Verification items for the finished model (mm, model axes). A direction names the side the tool comes from. Coordinates: 2 decimals unless noted, no trailing zeros. Order: outer loops, then holes, each group sorted by start corner. A loop starts at its lowest first (then second) coordinate and runs counter-clockwise, first axis right, second up. Notation, with made-up numbers: M -13.75,40 L 36.25,40 A14 cw 36.25,55 Z; hole C 53,75 d9. An arc over 180 degrees is marked long. Answer as a JSON object with one key per item and string values. Group by question number.
(1) Access from +Z, -Z, +X, -X, +Y, -Y to the whole of each face (thin tool, end or side, straight path). Record for faces 4 (the face through (38.1, -11, 37)), 5 (the face through (19, -14, 63.5)), 6 (the face through (39.39, -19.54, 53.44)).
(2) Mould release check, pull along Y, two halves, no side actions. Record for faces 1 (the face through (39.39, -6.84, 53.44)), 2 (the face through (-1.776, -0.724, 30.053)), 3 (the face through (-2.54, -14, 30)): released by +Y, released by -Y, zero draft, split by the parting line, or undercut.
(3) Material ranges on line 1 (X direction, y = -15.5, z = 17.5); line 2 (Y direction, x = 38.7, z = 54.61); line 3 (Y direction, x = 39, z = 54), recorded low to high.
(4) Cross-section at D-D (y = -6.35). Enter the section's corners in (x, z).
(5) Cross-section at A-A (z = 54.61). Count the separate pieces of the cut face and the enclosed holes in it, plus the area to 3 significant figures.
(6) Gauge pin test, flat ends, axial feed: pin 1 Ø1 at (x, z) = (23.5, 36) entering from +Y; pin 2 Ø7 at (x, y) = (14.5, -13.5) entering from -Z; pin 3 Ø4 at (x, y) = (19, -22.5) entering from -Z. Record the tip position at first contact, or that the pin passes through.
from build123d import *

# Parameters (mm, degrees)
BOSS_EXTRUDE2_DEPTH = 38.1
BOSS_EXTRUDE3_DEPTH = 2.54
BOSS_EXTRUDE5_START = 2.54
BOSS_EXTRUDE5_DEPTH = 2.54
FILLET1_R           = 2.54
FILLET3_R           = 2.54
FILLET5_R           = 2.54
SKETCH5_R           = 1.27
CUT_EXTRUDE1_DEPTH  = 2.54


with BuildPart() as part:
    # Sketch1 → Boss-Extrude2 (new body)
    with BuildSketch(Plane(origin=(0, 0, 0), x_dir=(0, 0, -1), z_dir=(1, 0, 0))):
        with BuildLine():
            Line((-60.96, 0), (-63.5, 0))
            Line((-63.5, 0), (-63.5, -25.4))
            Line((-63.5, -25.4), (-25.4, -25.4))
            ThreePointArc((-25.4, -25.4), (-7.439487758, -17.960512242), (0, 0))
            Line((0, 0), (-2.681549349, -2.54))
            ThreePointArc((-2.681549349, -2.54), (-10.16, -17.038837989), (-25.4, -22.86))
            Line((-25.4, -22.86), (-60.96, -22.86))
            Line((-60.96, -22.86), (-60.96, 0))
        make_face()
    extrude(amount=BOSS_EXTRUDE2_DEPTH)

    # Sketch2 → Boss-Extrude3 (add)
    with BuildSketch(Plane(origin=(38.1, 0, 0), x_dir=(0, 0, -1), z_dir=(1, 0, 0))):
        with BuildLine():
            Line((-63.5, 0), (0, 0))
            ThreePointArc((0, 0), (-7.439487758, -17.960512242), (-25.4, -25.4))
            Line((-25.4, -25.4), (-63.5, -25.4))
            Line((-63.5, -25.4), (-63.5, 0))
        make_face()
    extrude(amount=BOSS_EXTRUDE3_DEPTH)

    # Sketch3 → Boss-Extrude5 (add)
    with BuildSketch(Plane.ZY.offset(BOSS_EXTRUDE5_START)):
        with BuildLine():
            Line((2.681549349, -2.54), (0, 0))
            ThreePointArc((0, 0), (7.439487758, -17.960512242), (25.4, -25.4))
            Line((25.4, -25.4), (63.5, -25.4))
            Line((63.5, -25.4), (63.5, 0))
            Line((63.5, 0), (60.96, 0))
            Line((60.96, 0), (60.96, -22.86))
            Line((60.96, -22.86), (25.4, -22.86))
            ThreePointArc((25.4, -22.86), (10.16, -17.038837989), (2.681549349, -2.54))
        make_face()
        with BuildLine():
            Line((60.96, 0), (0, 0))
            Line((0, 0), (2.681549349, -2.54))
            ThreePointArc((2.681549349, -2.54), (10.16, -17.038837989), (25.4, -22.86))
            Line((25.4, -22.86), (60.96, -22.86))
            Line((60.96, -22.86), (60.96, 0))
        make_face()
    extrude(amount=-BOSS_EXTRUDE5_DEPTH)

    # Fillet1
    fillet1_edges = [part.edges().sort_by_distance(p)[0] for p in [
        (40.64, 0, 31.75),
    ]]
    fillet(fillet1_edges, radius=FILLET1_R - 0.0001)  # a hair under: the kernel refuses the full size

    # Fillet3
    fillet3_edges = [part.edges().sort_by_distance(p)[0] for p in [
        (-2.54, 0, 31.75),
    ]]
    fillet(fillet3_edges, radius=FILLET3_R - 0.0001)  # a hair under: the kernel refuses the full size

    # Fillet5
    fillet5_edges = [part.edges().sort_by_distance(p)[0] for p in [
        (40.64, -13.96995, 63.5),
        (39.896080514, -0.743919486, 63.5),
        (-2.54, -13.96995, 63.5),
        (-1.796080514, -0.743919486, 63.5),
        (19.05, 0, 63.5),
    ]]
    fillet(fillet5_edges, radius=FILLET5_R - 0.0001)  # a hair under: the kernel refuses the full size

    # Sketch5 → Cut-Extrude1 (cut)
    with BuildSketch(Plane(origin=(40.64, 0, 0), x_dir=(0, 0, -1), z_dir=(1, 0, 0))):
        with Locations((-54.61, -6.35)):
            Circle(SKETCH5_R)
        with Locations((-54.61, -19.05)):
            Circle(SKETCH5_R)
    extrude(amount=-CUT_EXTRUDE1_DEPTH, mode=Mode.SUBTRACT)


solid = part.part
Taken from the geometry:
{
 "1": {"face 4": "+Y", "face 5": "+Z, +X, -X, +Y, -Y", "face 6": "+X"},
 "2": {"face 1": "undercut", "face 2": "released by +Y", "face 3": "zero draft"},
 "3": {"line 1": "x = -2.54 to 0, 38.1 to 40.64", "line 2": "y = -25.4 to -20.32, -17.78 to -7.62, -5.08 to -0.07", "line 3": "y = -25.4 to -20.16, -17.94 to -7.46, -5.24 to -0.16"},
 "4": {"outline": "M -2.54,0.81 L 40.64,0.81 L 40.64,53.34 L 38.1,53.34 L 38.1,3.44 L 0,3.44 L 0,60.96 L 38.1,60.96 L 38.1,55.88 L 40.64,55.88 L 40.64,60.96 A2.54 ccw 38.1,63.5 L 0,63.5 A2.54 ccw -2.54,60.96 Z"},
 "5": {"separate pieces": "3", "enclosed holes": "0", "area": "210 mm²"},
 "6": {"pin 1": "stops at y = -22.86", "pin 2": "stops at z = 2.05", "pin 3": "stops at z = 10.4"}
}
